```python
from build123d import *

# Parameters (mm, degrees)
SKETCH1_R           = 12
BOSS_EXTRUDE1_DEPTH = 10
SKETCH2_R           = 12
SKETCH2_R_2         = 11.5
BOSS_EXTRUDE2_DEPTH = 4
SKETCH3_W           = 22
SKETCH3_H           = 20
BOSS_EXTRUDE3_DEPTH = 4
CHAMFER2_SIZE       = 0.5


with BuildPart() as part:
    # Sketch1 → Boss-Extrude1 (new body, symmetric)
    with BuildSketch(Plane(origin=(0, 0, 0), x_dir=(1, 0, 0), z_dir=(0, 1, 0))):
        with BuildLine():
            Line((15, -55), (-15, -55))
            Line((-15, -55), (-15, 0))
            ThreePointArc((-15, 0), (0, 15), (15, 0))
            Line((15, 0), (15, -55))
        make_face()
        Circle(SKETCH1_R, mode=Mode.SUBTRACT)
    extrude(amount=BOSS_EXTRUDE1_DEPTH, both=True)

    # Sketch2 → Boss-Extrude2 (add, symmetric)
    with BuildSketch(Plane(origin=(0, 0, 0), x_dir=(1, 0, 0), z_dir=(0, 1, 0))):
        Circle(SKETCH2_R)
        Circle(SKETCH2_R_2, mode=Mode.SUBTRACT)
    extrude(amount=BOSS_EXTRUDE2_DEPTH, both=True)

    # Sketch3 → Boss-Extrude3 (add)
    with BuildSketch(Plane.XY.offset(55)):
        Rectangle(SKETCH3_W, SKETCH3_H)
    extrude(amount=BOSS_EXTRUDE3_DEPTH)

    # Chamfer2
    chamfer2_edges = [part.edges().sort_by_distance(p)[0] for p in [
        (-15, 10, 27.5),
        (-12, -10, 0),
        (-12, 10, 0),
        (-13, 10, 55),
        (13, -10, 55),
        (13, 10, 55),
        (-11, 10, 57),
        (-11, -10, 57),
        (11, -10, 57),
        (11, 10, 57),
        (-11, 0, 59),
        (0, -10, 59),
        (11, 0, 59),
        (0, 10, 59),
        (15, 10, 27.5),
        (-13, -10, 55),
        (-15, -10, 27.5),
        (0, -10, -15),
        (15, -10, 27.5),
        (0, 10, -15),
        (15, 0, 55),
        (-15, 0, 55),
    ]]
    chamfer(chamfer2_edges, length=CHAMFER2_SIZE)


solid = part.part
```
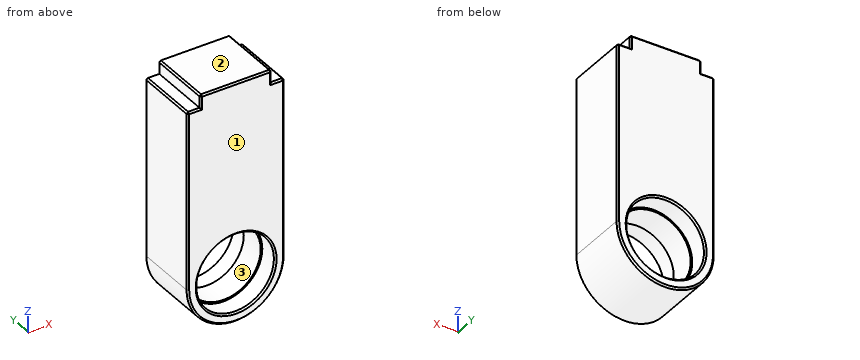
Input: part model. Units: mm. Frame: model coordinates. Face numbers are marked on the shaded views. Round coordinates to 2 decimals unless told otherwise and drop trailing zeros. Write each loop counter-clockwise with the first axis right and the second up, starting at its lowest first coordinate (ties: lowest second). Pieces come first, ordered by that corner, then holes. Notation, with made-up numbers: (-40, -2.75) - (-34, -2.75) arc R18 cw to (-34, 8.25) - close; hole circle Ø4 at (-40, -35). An arc over 180 degrees is marked (long way). Write item = value, one per line.
(1) Material intervals for probe 1 along Z at (x, y) = (0, 5.6); probe 2 along X at (y, z) = (-6, 56.5); probe 3 along X at (y, z) = (-1.5, 0), sorted ascending.
Geometry check:
probe_1 = -15 to -12, 12 to 59
probe_2 = -11 to 11
probe_3 = -15 to -11.5, 11.5 to 15
(2) Contact query for flat-ended pins moving along their axis: pin 1 Ø3 at (y, z) = (3, 57.5) entering from +X; pin 2 Ø5 at (x, y) = (-7, 1) entering from -Z; pin 3 Ø1 at (x, y) = (12, -3) entering from +Z. Output: stop coordinate, or through.
Geometry check:
pin_1 = 11
pin_2 = -14.31
pin_3 = 55
(3) Section query B-B on y = 8.5. Output: boundary loops of the cut face in (x, z).
Geometry check:
outline = (-15, 0) arc R15 ccw to (15, 0) - (15, 54.5) - (14.5, 55) - (11, 55) - (11, 58.5) - (10.5, 59) - (-10.5, 59) - (-11, 58.5) - (-11, 55) - (-14.5, 55) - (-15, 54.5) - close; hole circle Ø24 at (0, 0)
(4) Section query C-C on y = 2.75. Output: boundary loops of the cut face in (x, z), then the cut area to 3 significant figures.
Geometry check:
outline = (-15, 0) arc R15 ccw to (15, 0) - (15, 54.5) - (14.5, 55) - (11, 55) - (11, 58.5) - (10.5, 59) - (-10.5, 59) - (-11, 58.5) - (-11, 55) - (-14.5, 55) - (-15, 54.5) - close; hole circle Ø23 at (0, 0)
area = 1,680 mm^2
(5) Pull-direction query (Z, two-part tool) for the marked faces 1, 2 and 3; classes: +Z half, -Z half, draft (parallel to the pull), parting line (faces both ways), or undercut.
Geometry check:
face_1 = draft
face_2 = +Z half
face_3 = undercut
(6) Section query A-A on x = 0. Output: boundary loops of the cut face in (y, z).
Geometry check:
outline = (-10, -14.5) - (-9.5, -15) - (9.5, -15) - (10, -14.5) - (10, -12.5) - (9.5, -12) - (4, -12) - (4, -11.5) - (-4, -11.5) - (-4, -12) - (-9.5, -12) - (-10, -12.5) - close; (-10, 12.5) - (-9.5, 12) - (-4, 12) - (-4, 11.5) - (4, 11.5) - (4, 12) - (9.5, 12) - (10, 12.5) - (10, 58.5) - (9.5, 59) - (-9.5, 59) - (-10, 58.5) - close
